Study the drawing (mm; zero at the part's minimum x, y, z) and answer. A direction names the side the tool comes from. Give positions to 0.01 mm unless a question says otherwise; leave off trailing zeros. Order: outer loops, then holes, each group sorted by start corner. A loop starts at its lowest first (then second) coordinate and runs counter-clockwise, first axis right, second up.
Item 1: A cutting plane is placed at B-B (z = 10.75). Write down the section's boundary in (x, y), plus the area to 3 significant figures.
Item 2: A cutting plane is placed at A-A (y = 0.45). Write down the section's boundary in (x, z), plus the area to 3 significant figures.
Item 3: Which of the six approach directions +Z, -Z, +X, -X, +Y, -Y give full straight-line access (tool end or side, diameter ignored) to the marked faces 4 and 5?
Item 4: Given pin 1 Ø3.5 at (x, z) = (8, 9.5) entering from -Y, flat-ended and moving along its own axis, determine where the tip first touches the part or whether it passes through.
Item 5: The mould has two halves that part along Z. Classify the marked faces 1, 2 and 3: +Z half, -Z half, draft (parallel to the pull), parting line (faces both ways), or undercut.
Item 6: A cutting plane is placed at D-D (z = 15.25). Write down the section's boundary in (x, y), plus the area to 3 significant figures.
Item 7: A cutting plane is placed at C-C (x = 9.25). Write down the section's boundary in (y, z).
Item 8: Find the intervals of material crossed by line 1 along Z through (x, y) = (5.75, 0.3); line 2 along Y through (x, z) = (8, 11.75), in increasing order.
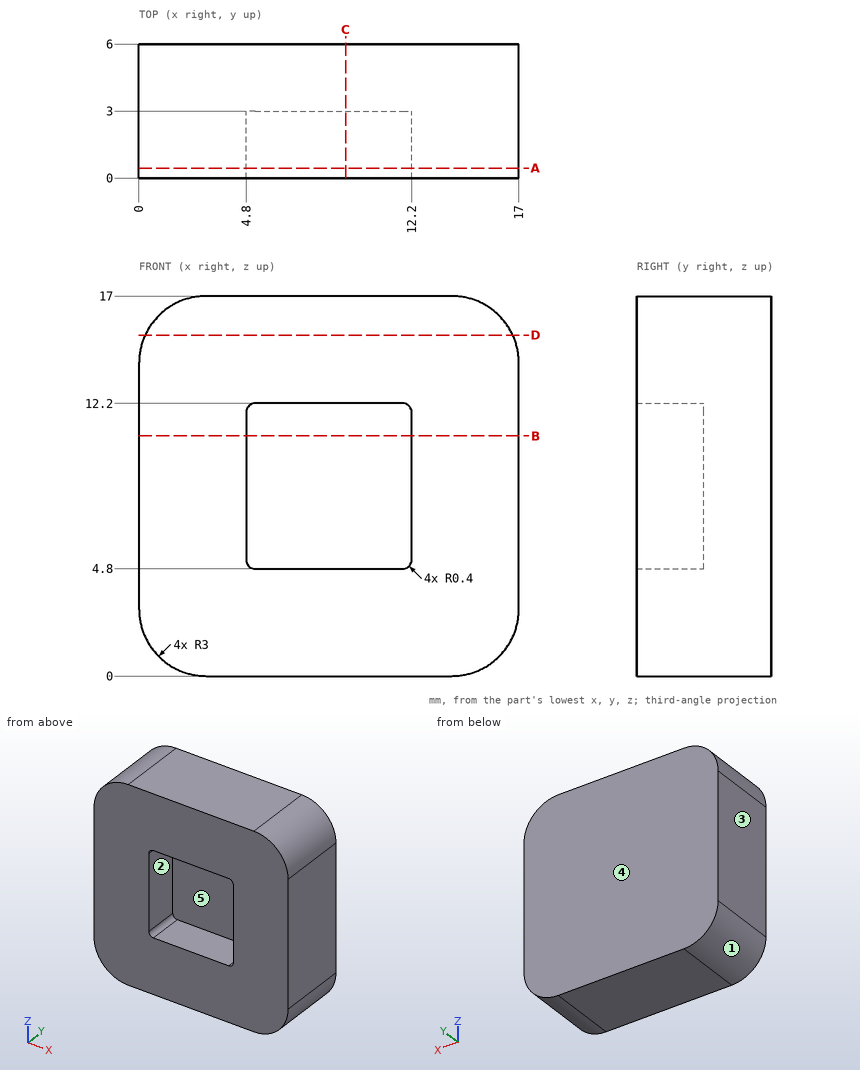
Response values:
1. outline: (0, 0) - (4.8, 0) - (4.8, 3) - (12.2, 3) - (12.2, 0) - (17, 0) - (17, 6) - (0, 6) - close
1. area: 79.8 mm2
2. outline: (0, 3) arc R3 ccw to (3, 0) - (14, 0) arc R3 ccw to (17, 3) - (17, 14) arc R3 ccw to (14, 17) - (3, 17) arc R3 ccw to (0, 14) - close; hole (4.8, 5.2) arc R0.4 ccw to (5.2, 4.8) - (11.8, 4.8) arc R0.4 ccw to (12.2, 5.2) - (12.2, 11.8) arc R0.4 ccw to (11.8, 12.2) - (5.2, 12.2) arc R0.4 ccw to (4.8, 11.8) - close
2. area: 227 mm2
3. face 4: +Z, -Z, +X, -X, +Y
3. face 5: -Y
4. pin 1: stops at y = 3
5. face 1: -Z half
5. face 2: undercut
5. face 3: draft
6. outline: (0.27, 0) - (16.73, 0) - (16.73, 6) - (0.27, 6) - close
6. area: 98.7 mm2
7. outline: (0, 0) - (6, 0) - (6, 17) - (0, 17) - (0, 12.2) - (3, 12.2) - (3, 4.8) - (0, 4.8) - close
8. line 1: z = 0 to 4.8, 12.2 to 17
8. line 2: y = 3 to 6
